Part print with two shaded views. Sizes in mm from the minimum x, y, z corner. Round coordinates to 2 decimals unless told otherwise and drop trailing zeros. Write each loop counter-clockwise with the first axis right and the second up, starting at its lowest first coordinate (ties: lowest second). Pieces come first, ordered by that corner, then holes.
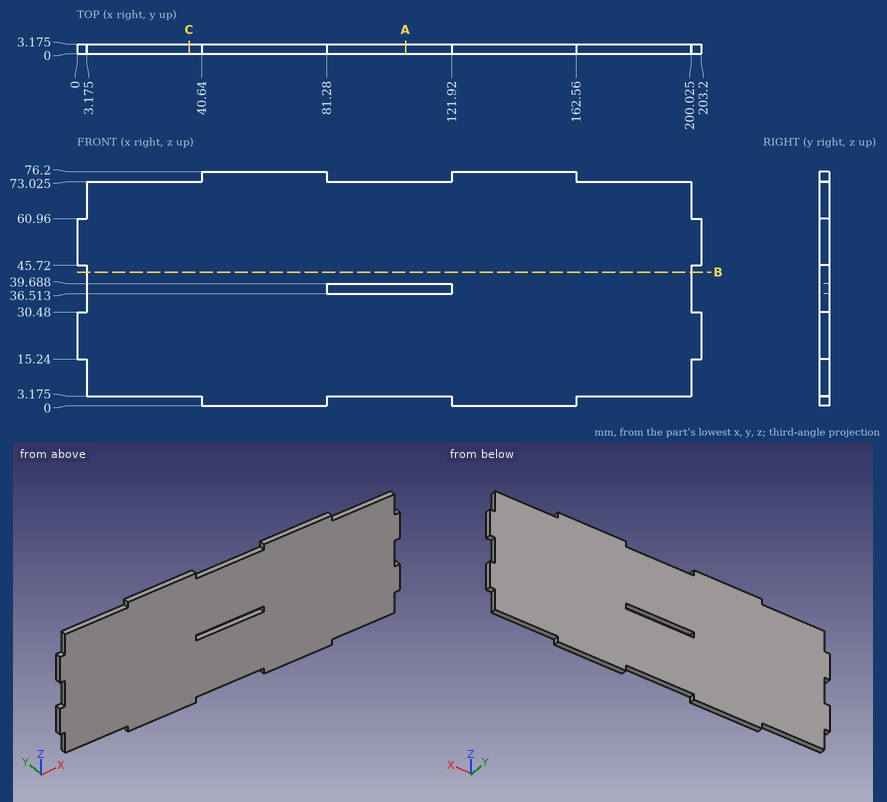
Q1. Cut at B-B on z = 43.5. Write the cut outline in (x, y) (1 decimal).
Values follow:
outline: (3.2, 0) - (200, 0) - (200, 3.2) - (3.2, 3.2) - close
Q2. Cut at A-A on x = 107. Write the cut outline in (y, z) (1 decimal).
Values follow:
outline: (0, 3.2) - (3.2, 3.2) - (3.2, 36.5) - (0, 36.5) - close; (0, 39.7) - (3.2, 39.7) - (3.2, 73) - (0, 73) - close
Q3. Wall check: L1, parallel to Z at x = 120, y = 2.75 (1 decimal); L2, parallel to X at y = 1.3, z = 11.5 (1 decimal); L3, parallel to Z at x = 183.5, y = 1.8 (1 decimal). Give the ranges that are in metal, low to high.
Values follow:
L1: z = 3.2 to 36.5, 39.7 to 73
L2: x = 3.2 to 200
L3: z = 3.2 to 73
Q4. Cut at C-C on x = 36.5. Write the cut outline in (y, z) (1 decimal), plus the area to 3 significant figures.
Values follow:
outline: (0, 3.2) - (3.2, 3.2) - (3.2, 73) - (0, 73) - close
area: 222 mm2
Q5. Drop flat-ended pins along their axis: pin 1 (1.6 mm diameter, centred on x = 201.5, y = 2, fed in from +Z); pin 2 (1 mm diameter, centred on x = 105.5, y = 1, fed in from -Z) (1 decimal); pin 3 (1 mm diameter, centred on y = 2, z = 1, fed in from -X). Give the stop position or say it passes through.
Values follow:
pin 1: stops at z = 60.96
pin 2: stops at z = 3.2
pin 3: stops at x = 40.64
